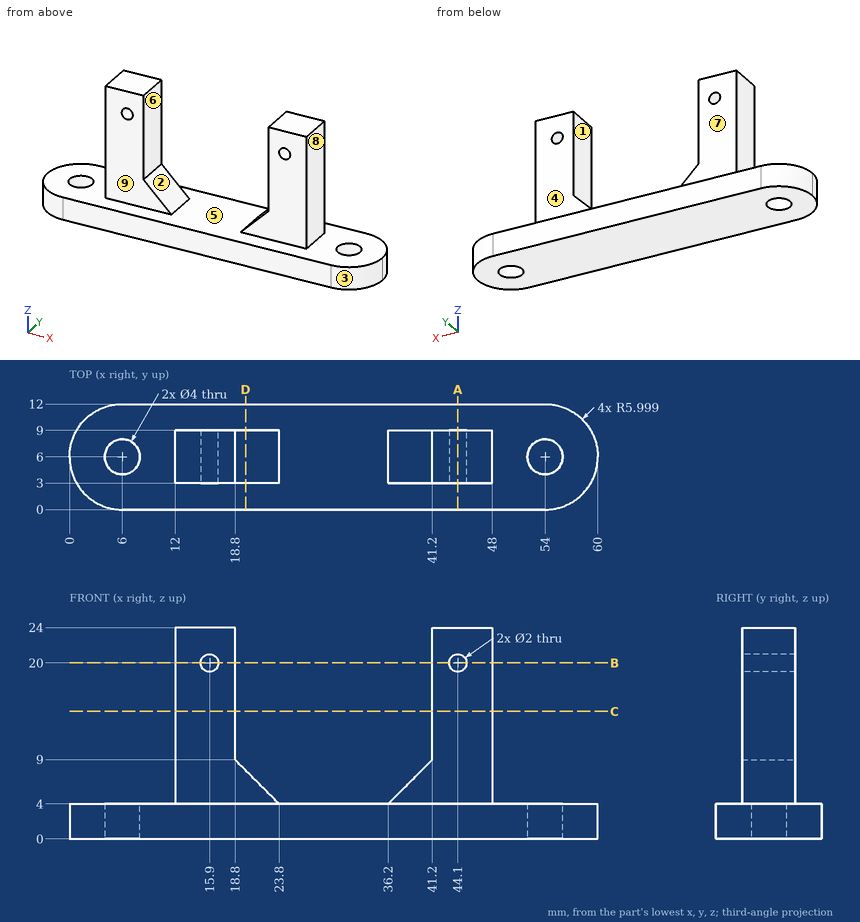
Job drawing, mm, ordinate dimensions from the low corner. One solid piece. A direction names the side the tool comes from. Coordinates: 2 decimals unless noted, no trailing zeros. Loops run counter-clockwise (first coordinate to the right, second up) from the corner with the lowest first, then second, coordinate; pieces in that order, holes last. Notation, with made-up numbers: (28, 60.5) -> (83, 60.5) arc R23 ccw to (83, 87.5) -> close; hole circle Ø6 at (-24, 46). An arc over 180 degrees is marked (long way). One line per item, written item: value.
1. Which spindle directions (+Z, -Z, +X, -X, +Y, -Y) get a long thin tool onto all of the face, cutting with end or side? Do the marked faces 5, 6, 7, 8 and 9. Say none if no direction does.
Answers:
face 5: +Z
face 6: +Z, +Y, -Y
face 7: +Z, +X, -X, +Y
face 8: +Z, +X, +Y, -Y
face 9: +Z, +X, -X, -Y
2. Slice it at D-D on x = 20. Write the cut outline in (y, z).
Answers:
outline: (0, 0) -> (12, 0) -> (12, 4) -> (9, 4) -> (9, 7.8) -> (3, 7.8) -> (3, 4) -> (0, 4) -> close
3. Slice it at A-A on x = 44.1. Write the cut outline in (y, z), and give its area (3 significant figures).
Answers:
outline: (0, 0) -> (12, 0) -> (12, 4) -> (9, 4) -> (9, 19) -> (3, 19) -> (3, 4) -> (0, 4) -> close; (3, 21) -> (9, 21) -> (9, 24) -> (3, 24) -> close
area: 156 mm^2
4. Pull direction X, two halves, no side cores. Call the marked faces 1, 2, 3 and 4: pulls with the +X half, pulls with the -X half, needs draft (parallel to the pull), parting line crosses it, or undercut.
Answers:
face 1: undercut
face 2: undercut
face 3: pulls with the +X half
face 4: needs draft
5. Drill centre lines: line 1 (X direction, y = 6, z = 1.1); line 2 (X direction, y = 4.7, z = 20); line 3 (Y direction, x = 54, z = 0.85). Where is each one in solid material? Low to high. Write a range as [from, to].
Answers:
line 1: x = [0, 4], [8, 52], [56, 60]
line 2: x = [12, 14.9], [16.9, 18.8], [41.2, 43.1], [45.1, 48]
line 3: y = [0, 4], [8, 12]
6. Flat gauge pins, fed straight in: P1, Ø3, axis at y = 7.5, z = 14.5, coming from the +X side; P2, Ø6.5, axis at x = 6, y = 6, coming from the +Z side; P3, Ø1.8, axis at y = 7, z = 17, coming from the -X side. Where does each tip first touch, or does it go through?
Answers:
P1: stops at x = 48
P2: stops at z = 4
P3: stops at x = 12
7. Slice it at C-C on z = 14.5. Write the cut outline in (x, y).
Answers:
outline: (12, 3) -> (18.8, 3) -> (18.8, 9) -> (12, 9) -> close; (41.2, 3) -> (48, 3) -> (48, 9) -> (41.2, 9) -> close
8. Slice it at B-B on z = 20. Write the cut outline in (x, y), and give its area (3 significant figures).
Answers:
outline: (12, 3) -> (14.9, 3) -> (14.9, 9) -> (12, 9) -> close; (16.9, 3) -> (18.8, 3) -> (18.8, 9) -> (16.9, 9) -> close; (41.2, 3) -> (43.1, 3) -> (43.1, 9) -> (41.2, 9) -> close; (45.1, 3) -> (48, 3) -> (48, 9) -> (45.1, 9) -> close
area: 57.6 mm^2
